Geometry check sheet. Reference: the model listing, model coordinates, mm. A direction names the side the tool comes from. Coordinates: 2 decimals unless noted, no trailing zeros. Order: outer loops, then holes, each group sorted by start corner. A loop starts at its lowest first (then second) coordinate and runs counter-clockwise, first axis right, second up. Notation, with made-up numbers: (-38, 67) - (11, 67) arc R24 cw to (11, 77) - close; hole circle Ø2 at (18, 81). An arc over 180 degrees is marked (long way). Return JSON: item names as keys, results as strings. Group by question number.
Item 1: Section check B-B on x = 57.5. Give the number of separate pieces and of enclosed holes in the cut face, then the cut area to 3 significant figures.
Item 2: Tool access check on faces 1 (the flat face through (-13.537, -44.151, 26.79)), 2 (the flat face through (10.112, 86, 20)), 3 (the flat face through (-85.92, -8.05, 22.83)), 4 (the flat face through (-61.1, 27.9, 47)), 5 (the cylindrical face through (-54.09, 56.2, 19.6)). Record the directions out of +Z, -Z, +X, -X, +Y, -Y that give a thin tool (end or side, any length) a straight path to the whole face; none if there is none.
Item 3: Section check A-A on z = -77. Enter the section's corners in (x, y).
Item 4: Draft check along Z on faces 6 (the cylindrical face through (0.651, 62.457, -97.605)), 7 (the flat face through (-27, -38, 42)), 8 (the flat face through (89, -1, 8)), 9 (the cylindrical face through (0.554, 74.998, -45.63)). Enter one of: pulls with the +Z half, pulls with the -Z half, needs draft (parallel to the pull), parting line crosses it, or undercut.
Item 5: Gauge pin test, flat ends, axial feed: pin 1 (4.5 mm diameter, centred on x = -6.5, y = 46.5, fed in from +Z); pin 2 (16 mm diameter, centred on x = 0, y = -57.5, fed in from +Z); pin 3 (5 mm diameter, centred on x = -87, z = 26, fed in from +Y); pin 4 (13.5 mm diameter, centred on x = 0, y = 0, fed in from +Z). Record the tip position at first contact, or that the pin passes through.
Item 6: Scan lines: probe 1 along Y at (x, z) = (0, -101.75); probe 2 along Z at (x, y) = (57, -16); probe 3 along Z at (x, y) = (-68, 20). Record each from-to range of solid material in increasing order.
from build123d import *
from build123d.topology import SkipClean

# Parameters (mm, degrees)
SKETCH1_R           = 85
BOSS_EXTRUDE1_DEPTH = 10
SKETCH4_R           = 74.5
BOSS_EXTRUDE2_DEPTH = 15
SKETCH5_R           = 67
CUT_EXTRUDE1_DEPTH  = 20
SKETCH6_R           = 78
CUT_EXTRUDE2_DEPTH  = 15
BOSS_EXTRUDE3_DEPTH = 24
CIRPATTERN1_COUNT   = 4
CIRPATTERN2_COUNT   = 4
SKETCH14_R          = 17
BOSS_EXTRUDE4_DEPTH = 15
SKETCH15_R          = 11.3
CUT_EXTRUDE3_DEPTH  = 6
SKETCH16_R          = 7.5
CUT_EXTRUDE4_DEPTH  = 138.676917333
BOSS_EXTRUDE5_DEPTH = 30
BOSS_EXTRUDE6_START = 90
BOSS_EXTRUDE6_DEPTH = 90
BOSS_EXTRUDE7_START = 15
SKETCH19_R          = 85
BOSS_EXTRUDE7_DEPTH = 15
SKETCH20_R          = 47.5
CUT_EXTRUDE5_DEPTH  = 15
SKETCH21_R          = 5
CUT_EXTRUDE6_DEPTH  = 15
CIRPATTERN3_COUNT   = 4
SKETCH22_R          = 16.5
CUT_EXTRUDE7_DEPTH  = 9
FILLET1_R           = 5
SKETCH23_R          = 44
CUT_EXTRUDE8_DEPTH  = 5


with BuildPart() as part:
    # Sketch1 → Boss-Extrude1 (new body)
    with BuildSketch(Plane.XY):
        Circle(SKETCH1_R)
    extrude(amount=BOSS_EXTRUDE1_DEPTH)

    # Loft1: read off the stored shape, not the designer's step
    # Loft1: loft between two sections, ruled curve by curve
    loft1_from = [
        Edge.make_bspline([(-84.985889817, -1.548719476, 10), (-81.888450866, -171.52049911, 10), (88.083328768, -168.423060158, 10), (84.985889817, 1.548719476, 10), (81.888450866, 171.52049911, 10), (-88.083328768, 168.423060158, 10), (-84.985889817, -1.548719476, 10)], [0, 0, 0, 0, 0.5, 0.5, 0.5, 1, 1, 1, 1], 3, [1, 0.333333333, 0.333333333, 1, 0.333333333, 0.333333333, 1]),
    ]
    loft1_to = [
        Edge.make_bspline([(-77.561105187, -19.602932488, 32), (-38.35524021, -174.725142863, 32), (116.766970164, -135.519277886, 32), (77.561105187, 19.602932488, 32), (38.35524021, 174.725142863, 32), (-116.766970164, 135.519277886, 32), (-77.561105187, -19.602932488, 32)], [0, 0, 0, 0, 0.5, 0.5, 0.5, 1, 1, 1, 1], 3, [1, 0.333333333, 0.333333333, 1, 0.333333333, 0.333333333, 1]),
    ]
    loft1 = Solid(Shell([*[Face.make_surface_from_curves(loft1_from[k], loft1_to[k]) for k in range(1)], Face(Wire(loft1_from)), Face(Wire(loft1_to))]))
    add(loft1)

    # Sketch4 → Boss-Extrude2 (add)
    with BuildSketch(Plane.XY.offset(32)):
        Circle(SKETCH4_R)
    extrude(amount=BOSS_EXTRUDE2_DEPTH)

    # Sketch5 → Cut-Extrude1 (cut)
    with BuildSketch(Plane.XY.offset(47)):
        Circle(SKETCH5_R)
    extrude(amount=-CUT_EXTRUDE1_DEPTH, mode=Mode.SUBTRACT)

    # Sketch6 → Cut-Extrude2 (cut)
    with BuildSketch(Plane.XY.offset(27)):
        Circle(SKETCH6_R)
    extrude(amount=-CUT_EXTRUDE2_DEPTH, mode=Mode.SUBTRACT)

    # Sketch7 → Boss-Extrude3 (add)
    with BuildSketch(Plane.XY.offset(32)):
        with BuildLine():
            Line((10.112026185, 72.868932946), (10.112026185, 89.597937942))
            ThreePointArc((10.112026185, 89.597937942), (1.241313299, 95.599557722), (-7.797588157, 89.854364291))
            Line((-7.797588157, 89.854364291), (-8.860692334, 73.2984328))
            Line((-8.860692334, 73.2984328), (10.112026185, 72.868932946))
        make_face()
    boss_extrude3 = extrude(amount=-BOSS_EXTRUDE3_DEPTH)

    # CirPattern1: Boss-Extrude3 ×4 about axis
    cirpattern1_axis = Axis((0, 0, 0), (0, 0, 1))
    for i in range(1, CIRPATTERN1_COUNT):
        add(boss_extrude3.rotate(cirpattern1_axis, i * 360 / CIRPATTERN1_COUNT))

    # Sketch13 → M12x1.25 Tapped Hole1 (revolve, cut)
    with BuildSketch(Plane(origin=(0, 87, 32), x_dir=(0, -1, 0), z_dir=(1, 0, 0))):
        Polygon((0, 0), (0, 23.494647343), (5.4, 20.25), (5.4, 0), align=None)
    m12x1_25_tapped_hole1 = revolve(axis=Axis((0, 87, 38.35), (0, 0, -1)), mode=Mode.SUBTRACT)

    # CirPattern2: M12x1.25 Tapped Hole1 ×4 about axis
    cirpattern2_axis = Axis((0, 0, 0), (0, 0, 1))
    for i in range(1, CIRPATTERN2_COUNT):
        add(m12x1_25_tapped_hole1.rotate(cirpattern2_axis, i * 360 / CIRPATTERN2_COUNT), mode=Mode.SUBTRACT)

    # Sketch14 → Boss-Extrude4 (add)
    with BuildSketch(Plane.XY.offset(12)):
        Circle(SKETCH14_R)
    extrude(amount=BOSS_EXTRUDE4_DEPTH)

    # Sketch15 → Cut-Extrude3 (cut)
    with BuildSketch(Plane.XY.offset(27)):
        Circle(SKETCH15_R)
    extrude(amount=-CUT_EXTRUDE3_DEPTH, mode=Mode.SUBTRACT)

    # Sketch16 → Cut-Extrude4 (cut, through all)
    with BuildSketch(Plane.XY.offset(21)):
        Circle(SKETCH16_R)
    extrude(amount=-CUT_EXTRUDE4_DEPTH, mode=Mode.SUBTRACT)

    # Sketch17 → Boss-Extrude5 (add)
    with BuildSketch(Plane.XY.offset(12)):
        with BuildLine():
            Line((33.183444972, 26.553888224), (40.727249767, 29.005018986))
            ThreePointArc((40.727249767, 29.005018986), (47.552825815, 15.450849719), (49.997759598, 0.473323497))
            Line((49.997759598, 0.473323497), (42.453954803, -1.977807265))
            ThreePointArc((42.453954803, -1.977807265), (40.419901943, 13.133222261), (33.183444972, 26.553888224))
        make_face()
        with BuildLine():
            Line((15, 39.764934301), (15, 47.696960071))
            ThreePointArc((15, 47.696960071), (0, 50), (-15, 47.696960071))
            Line((-15, 47.696960071), (-15, 39.764934301))
            ThreePointArc((-15, 39.764934301), (0, 42.5), (15, 39.764934301))
        make_face()
        with BuildLine():
            Line((35.508496856, -23.353728846), (40.170824624, -29.770872493))
            ThreePointArc((40.170824624, -29.770872493), (29.389262615, -40.450849719), (15.900314793, -47.404430062))
            Line((15.900314793, -47.404430062), (11.237987025, -40.987286414))
            ThreePointArc((11.237987025, -40.987286414), (24.980873222, -34.383222261), (35.508496856, -23.353728846))
        make_face()
        with BuildLine():
            Line((-11.237987025, -40.987286414), (-15.900314793, -47.404430062))
            ThreePointArc((-15.900314793, -47.404430062), (-29.389262615, -40.450849719), (-40.170824624, -29.770872493))
            Line((-40.170824624, -29.770872493), (-35.508496856, -23.353728846))
            ThreePointArc((-35.508496856, -23.353728846), (-24.980873222, -34.383222261), (-11.237987025, -40.987286414))
        make_face()
        with BuildLine():
            Line((-42.453954803, -1.977807265), (-49.997759598, 0.473323497))
            ThreePointArc((-49.997759598, 0.473323497), (-47.552825815, 15.450849719), (-40.727249767, 29.005018986))
            Line((-40.727249767, 29.005018986), (-33.183444972, 26.553888224))
            ThreePointArc((-33.183444972, 26.553888224), (-40.419901943, 13.133222261), (-42.453954803, -1.977807265))
        make_face()
    extrude(amount=BOSS_EXTRUDE5_DEPTH)

    # Sketch18 → Boss-Extrude6 (add)
    with SkipClean():  # the faces are left unmerged after this step: merging them gives an invalid solid
        with BuildSketch(Plane(origin=(0, 0, 0), x_dir=(-1, 0, 0), z_dir=(0, 0, -1)).offset(BOSS_EXTRUDE6_START)):
            with BuildLine():
                Line((37.739875069, 64.812821492), (42.771858411, 73.454531025))
                ThreePointArc((42.771858411, 73.454531025), (0, 85), (-42.771858411, 73.454531025))
                Line((-42.771858411, 73.454531025), (-37.739875069, 64.812821492))
                ThreePointArc((-37.739875069, 64.812821492), (0, 75), (37.739875069, 64.812821492))
            make_face()
            with BuildLine():
                Line((37.739875069, -64.812821492), (42.771858411, -73.454531025))
                ThreePointArc((42.771858411, -73.454531025), (0, -85), (-42.771858411, -73.454531025))
                Line((-42.771858411, -73.454531025), (-37.739875069, -64.812821492))
                ThreePointArc((-37.739875069, -64.812821492), (0, -75), (37.739875069, -64.812821492))
            make_face()
        extrude(amount=-BOSS_EXTRUDE6_DEPTH)

    # Sketch19 → Boss-Extrude7 (add)
    with BuildSketch(Plane(origin=(0, 0, -90), x_dir=(-1, 0, 0), z_dir=(0, 0, -1)).offset(BOSS_EXTRUDE7_START)):
        Circle(SKETCH19_R)
    extrude(amount=-BOSS_EXTRUDE7_DEPTH)

    # Sketch20 → Cut-Extrude5 (cut)
    with BuildSketch(Plane(origin=(0, 0, -105), x_dir=(-1, 0, 0), z_dir=(0, 0, -1))):
        Circle(SKETCH20_R)
    extrude(amount=-CUT_EXTRUDE5_DEPTH, mode=Mode.SUBTRACT)

    # Sketch21 → Cut-Extrude6 (cut)
    with BuildSketch(Plane(origin=(0, 0, -105), x_dir=(-1, 0, 0), z_dir=(0, 0, -1))):
        with Locations((0, 57.5)):
            Circle(SKETCH21_R)
    cut_extrude6 = extrude(amount=-CUT_EXTRUDE6_DEPTH, mode=Mode.SUBTRACT)

    # CirPattern3: Cut-Extrude6 ×4 about axis
    cirpattern3_axis = Axis((0, 0, 0), (0, 0, 1))
    for i in range(1, CIRPATTERN3_COUNT):
        add(cut_extrude6.rotate(cirpattern3_axis, i * 360 / CIRPATTERN3_COUNT), mode=Mode.SUBTRACT)

    # Sketch22 → Cut-Extrude7 (cut)
    with BuildSketch(Plane(origin=(0, 0, 0), x_dir=(-1, 0, 0), z_dir=(0, 0, -1))):
        Circle(SKETCH22_R)
    extrude(amount=-CUT_EXTRUDE7_DEPTH, mode=Mode.SUBTRACT)

    # Fillet1
    fillet1_edges = [part.edges().sort_by_distance(p)[0] for p in [
        (16.5, 0, 9),
    ]]
    fillet(fillet1_edges, radius=FILLET1_R)

    # Sketch23 → Cut-Extrude8 (cut)
    with SkipClean():  # the faces are left unmerged after this step: merging them gives an invalid solid
        with BuildSketch(Plane.XY.offset(42)):
            Circle(SKETCH23_R)
        extrude(amount=-CUT_EXTRUDE8_DEPTH, mode=Mode.SUBTRACT)


solid = part.part
Computed:
{
 "1": {"separate pieces": "3", "enclosed holes": "0", "area": "4,020 mm²"},
 "2": {"face 1": "+Z", "face 2": "+Z, +X, +Y", "face 3": "+Z, -X, -Y", "face 4": "+Z, +X, -X, +Y, -Y", "face 5": "none"},
 "3": {"outline": "(-42.77, -73.45) arc R85 ccw to (42.77, -73.45) - (37.74, -64.81) arc R75 cw to (-37.74, -64.81) - close; (-42.77, 73.45) - (-37.74, 64.81) arc R75 cw to (37.74, 64.81) - (42.77, 73.45) arc R85 ccw to start"},
 "4": {"face 6": "needs draft", "face 7": "pulls with the +Z half", "face 8": "pulls with the -Z half", "face 9": "undercut"},
 "5": {"pin 1": "stops at z = 42", "pin 2": "stops at z = 12", "pin 3": "stops at y = 10.11", "pin 4": "passes through"},
 "6": {"probe 1": "y = -85 to -62.5, -52.5 to -47.5, 47.5 to 52.5, 62.5 to 85", "probe 2": "z = -105 to -90, 0 to 12", "probe 3": "z = -105 to -90, 0 to 12, 27 to 47"}
}
